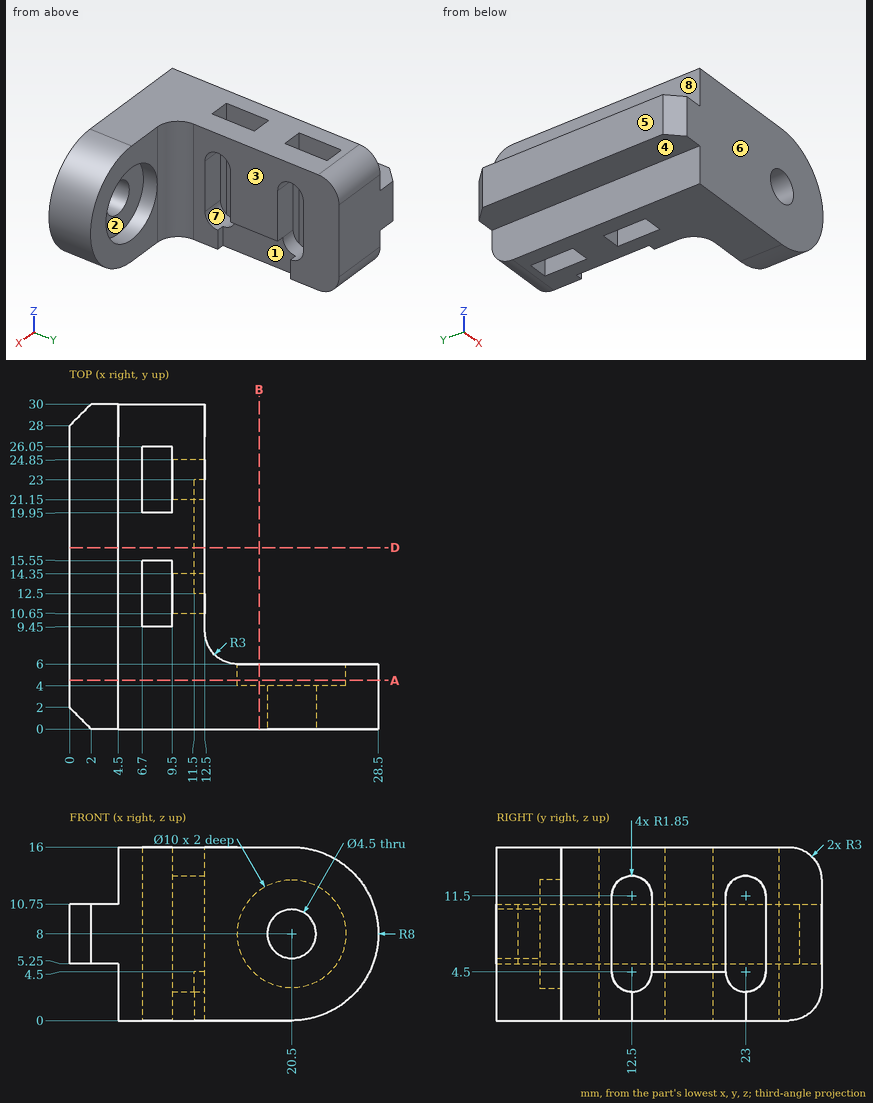
For this review, use the dimensioned drawing (mm, ordinates from the lowest corner) and the shaded views. A direction names the side the tool comes from. Round coordinates to 2 decimals unless told otherwise and drop trailing zeros. Write each loop counter-clockwise with the first axis right and the second up, starting at its lowest first coordinate (ties: lowest second). Pieces come first, ordered by that corner, then holes. Notation, with made-up numbers: (84.5, 43) - (113.5, 43) arc R16 cw to (113.5, 55) - close; hole circle Ø9 at (-4.5, 62). An arc over 180 degrees is marked (long way). One line per item, written item: value. Start each with the question number.
1. Consider section B-B on x = 17.5. Write out the cut boundary in (y, z).
2. Machinability: for the marked faces 1, 2, 3, 4 and 5, which of the approach directions +Z, -Z, +X, -X, +Y, -Y give a long, thin tool a straight path to every point of the face, cutting with its end or side? Answer none if there is none.
3. The part is to be moulded in two halves that separate along Y. For the marked faces 6, 7 and 8, say which applies: released by +Y, released by -Y, zero draft, split by the parting line, or undercut.
4. Consider section A-A on y = 4.5. Write out the cut boundary in (x, z), and give its area (3 significant figures).
5. Clearance check with flat-ended pins moving along their axes: P1, Ø8, axis at x = 20.5, z = 8, coming from the +Y side; P2, Ø2, axis at x = 3, y = 9, coming from the -Z side; P3, Ø1.8, axis at y = 12, z = 11.5, coming from the +X side. State where each tip first meets the part, or that it passes through.
6. To check wall thickness, follow L1, parallel to Z at x = 20.5, y = 4.5; L2, parallel to X at y = 3, z = 8; L3, parallel to X at y = 24, z = 15. State the ranges of each line that lie inside material, in increasing order. Write a range as from..to.
7. Consider section D-D on y = 16.75. Write out the cut boundary in (x, z), and give its area (3 significant figures).
Checks:
1. outline: (0, 0) - (6, 0) - (6, 4) - (4, 4) - (4, 12) - (6, 12) - (6, 16) - (0, 16) - close
2. face 1: -Z, +X
2. face 2: +Y
2. face 3: +Z, -Z, +X, +Y
2. face 4: -Z, -X, +Y, -Y
2. face 5: +Z, -Z, -X, +Y, -Y
3. face 6: released by -Y
3. face 7: undercut
3. face 8: zero draft
4. outline: (0, 5.25) - (4.5, 5.25) - (4.5, 0) - (20.5, 0) arc R8 ccw to (20.5, 16) - (4.5, 16) - (4.5, 10.75) - (0, 10.75) - close; hole circle Ø10 at (20.5, 8)
4. area: 303 mm^2
5. P1: stops at y = 4
5. P2: stops at z = 5.25
5. P3: stops at x = 6.7
6. L1: z = 0..3, 13..16
6. L2: x = 0..18.25, 22.75..28.5
6. L3: x = 4.5..6.7, 9.5..12.5
7. outline: (0, 5.25) - (4.5, 5.25) - (4.5, 0) - (11.5, 0) - (11.5, 4.5) - (12.5, 4.5) - (12.5, 16) - (4.5, 16) - (4.5, 10.75) - (0, 10.75) - close
7. area: 148 mm^2
